Could you check a few things on this drawing? It's one solid part, dimensions in mm from its lowest x, y, z. A direction names the side the tool comes from. Give positions to 0.01 mm unless a question says otherwise; leave off trailing zeros. Order: outer loops, then holes, each group sorted by start corner. A loop starts at its lowest first (then second) coordinate and runs counter-clockwise, first axis right, second up.
Item 1: I want a section at A-A, the plane x = 44. Write out the boundary of the cut face in (y, z), then the cut area to 3 significant figures.
Item 2: I'm going to push flat-ended pins straight in: pin 1 Ø21 at (y, z) = (27, 29) entering from +X; pin 2 Ø24 at (x, z) = (40.5, 37.5) entering from +Y; pin 3 Ø1.5 at (y, z) = (14, 23) entering from +X. Where does each tip first touch, or does it pass through?
Item 3: If we mould it in two halves opening along X, with no side actions, what happens to the marked faces 5, 6 and 7? For each: +X half, -X half, draft (parallel to the pull), parting line (faces both ways), or undercut.
Item 4: I want a section at D-D, the plane y = 11.5. Write out the boundary of the cut face in (x, z), then the cut area to 3 significant figures.
Item 5: I want a section at C-C, the plane x = 8.5. Write out the boundary of the cut face in (y, z).
Item 6: Which directions (+Z, -Z, +X, -X, +Y, -Y) give clear straight access to the entire face, cutting with the end or side of a thin tool? Please do the marked faces 1, 2, 3 and 4.
Item 7: If I drill on line 1 along X through (y, z) = (2.5, 8.5); line 2 along Z through (x, y) = (34, 20); line 3 along X through (y, z) = (20, 33.5), over which ranges is the centre line in solid material (lowest first)?
Item 8: I want a section at B-B, the plane z = 29. Write out the boundary of the cut face in (x, y), then the cut area to 3 significant figures.
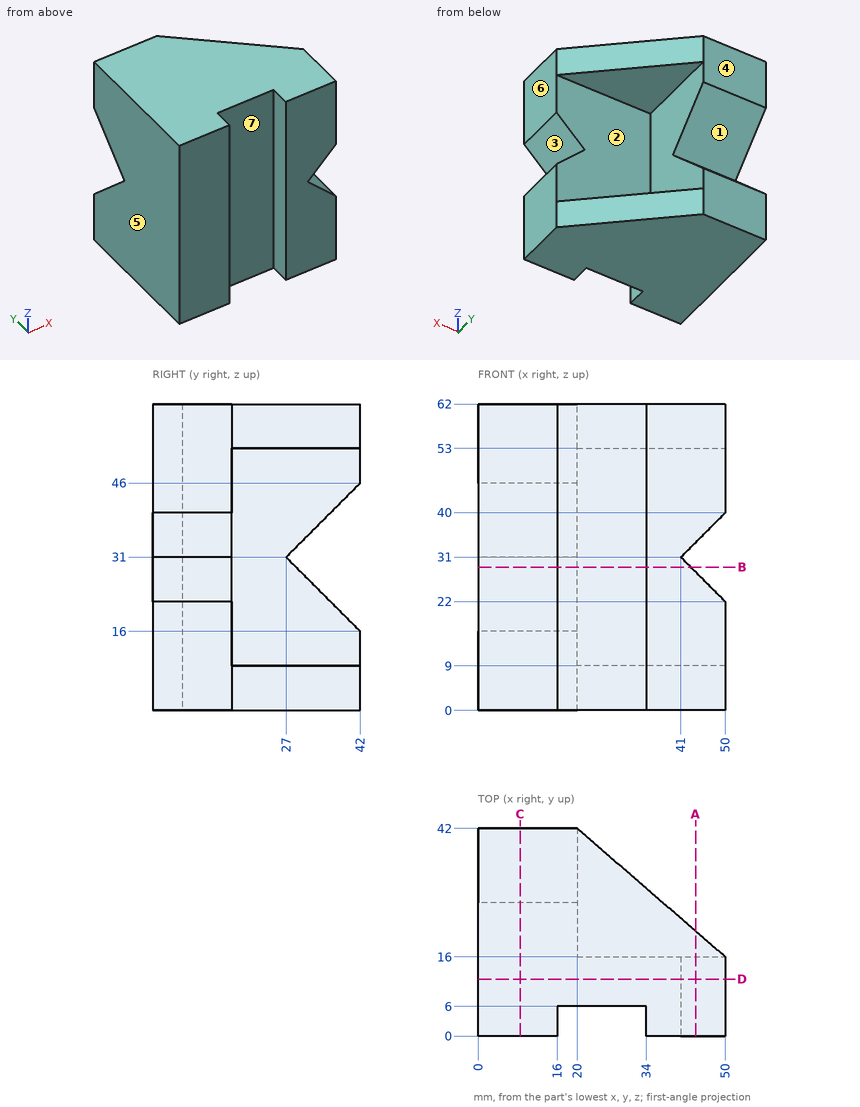
Results list:
1. outline: (0, 0) - (21.2, 0) - (21.2, 9) - (16, 9) - (16, 28) - (0, 28) - close; (0, 34) - (16, 34) - (16, 53) - (21.2, 53) - (21.2, 62) - (0, 62) - close
1. area: 990 mm2
2. pin 1: stops at x = 20
2. pin 2: stops at y = 16
2. pin 3: stops at x = 49.75
3. face 5: -X half
3. face 6: +X half
3. face 7: undercut
4. outline: (0, 0) - (50, 0) - (50, 22) - (41, 31) - (50, 40) - (50, 62) - (0, 62) - close
4. area: 3,020 mm2
5. outline: (0, 0) - (42, 0) - (42, 16) - (27, 31) - (42, 46) - (42, 62) - (0, 62) - close
6. face 1: +X, -X, +Y
6. face 2: +X, +Y
6. face 3: +X, +Y, -Y
6. face 4: +Z, -Z, +X, -X, +Y
7. line 1: x = 0 to 16, 34 to 50
7. line 2: z = 0 to 9, 53 to 62
7. line 3: x = 0 to 20
8. outline: (0, 0) - (16, 0) - (16, 6) - (34, 6) - (34, 0) - (43, 0) - (43, 16) - (20, 16) - (20, 29) - (0, 29) - close
8. area: 840 mm2
